The model under review builds one solid part; all positions refer to its coordinate system, in mm. A direction names the side the tool comes from. Round coordinates to 2 decimals unless told otherwise and drop trailing zeros. Order: outer loops, then holes, each group sorted by start corner. A loop starts at its lowest first (then second) coordinate and runs counter-clockwise, first axis right, second up. Notation, with made-up numbers: (54, -12.5) -> (108, -12.5) arc R7 cw to (108, -2.5) -> close; hole circle Ø9 at (-14.75, 34). An arc over 180 degrees is marked (long way). Put each result on its own line as item: value. Start each with the question number.
from build123d import *

# Parameters (mm, degrees)
F0_W     = 73
F0_H     = 60
F0_W_2   = 13
F0_H_2   = 15
F0_R     = 1.6
F1_DEPTH = 3
F2_R     = 1


with BuildPart() as f1:
    # F0 (on Top) → F1 (new body)
    with BuildSketch(Plane.XY):
        with Locations((-36.5, -30)):
            Rectangle(F0_W, F0_H)
        with Locations((-63, -49)):
            Rectangle(F0_W_2, F0_H_2, mode=Mode.SUBTRACT)
        with Locations((-50.948029, -30)):
            Circle(F0_R, mode=Mode.SUBTRACT)
        with Locations((-28.448029, -30)):
            Circle(F0_R, mode=Mode.SUBTRACT)
    extrude(amount=F1_DEPTH)

    # F2
    f2_edges = [f1.edges().sort_by_distance(p)[0] for p in [
        (-69.5, -41.5, 1.5),
        (-56.5, -56.5, 1.5),
        (-69.5, -56.5, 1.5),
        (-56.5, -41.5, 1.5),
    ]]
    fillet(f2_edges, radius=F2_R)


solid = f1.part
Q1. Take a section at C-C on x = -50.5. Give the boundary of the cut face in (y, z).
Q2. Take a section at B-B on z = 0.7. Give the boundary of the cut face in (x, y), and give its area (3 significant figures).
Q3. Draft analysis for pull direction X (two halves, no side actions). For faces 3 (the face through (0, -30, 1)), 4 (the face through (-63, -56.5, 1)), 5 (the face through (-37, -60, 1)), state which applies: +X half, -X half, draft (parallel to the pull), parting line (faces both ways), or undercut.
Q4. For faces 1 (the face through (-37, 0, 1)), 2 (the face through (-69.5, -49, 1)), list the 3-axis set-ups (+Z, -Z, +X, -X, +Y, -Y) from which the entire face can be reached by the end or side of a thin tool; tool diameter is ignored.
Q5. Wall thickness on probe 1 along X at (y, z) = (-53, 1.45); probe 2 along Y at (x, z) = (-28.5, 2.2); probe 3 along Y at (x, z) = (-62.5, 2.1): over which ranges is each line inside the solid? List them lowest first. Write a range as [from, to].
Q6. Clearance check with a flat-ended pin moving along its axis: pin 1 Ø3 at (x, y) = (-28.45, -30) entering from +Z. State where the tip first meets the part, or that it passes through.
Q7. Take a section at A-A on y = -30. Give the boundary of the cut face in (x, z), and give its area (3 significant figures).
Calculated:
1. outline: (-60, 0) -> (-31.54, 0) -> (-31.54, 3) -> (-60, 3) -> close; (-28.46, 0) -> (0, 0) -> (0, 3) -> (-28.46, 3) -> close
2. outline: (-73, -60) -> (0, -60) -> (0, 0) -> (-73, 0) -> close; hole (-69.5, -55.5) arc R1 ccw to (-68.5, -56.5) -> (-57.5, -56.5) arc R1 ccw to (-56.5, -55.5) -> (-56.5, -42.5) arc R1 ccw to (-57.5, -41.5) -> (-68.5, -41.5) arc R1 ccw to (-69.5, -42.5) -> close; hole circle Ø3.2 at (-50.95, -30); hole circle Ø3.2 at (-28.45, -30)
2. area: 4,170 mm²
3. face 3: +X half
3. face 4: undercut
3. face 5: draft
4. face 1: +Z, -Z, +X, -X, +Y
4. face 2: +Z, -Z
5. probe 1: x = [-73, -69.5], [-56.5, 0]
5. probe 2: y = [-60, -31.6], [-28.4, 0]
5. probe 3: y = [-60, -56.5], [-41.5, 0]
6. pin 1: passes through
7. outline: (-73, 0) -> (-52.55, 0) -> (-52.55, 3) -> (-73, 3) -> close; (-49.35, 0) -> (-30.05, 0) -> (-30.05, 3) -> (-49.35, 3) -> close; (-26.85, 0) -> (0, 0) -> (0, 3) -> (-26.85, 3) -> close
7. area: 200 mm²
